Here's how the part is built. I have some questions about the finished solid (model axes, mm). Face numbers are marked on the shaded views. Give positions to 0.01 mm unless a question says otherwise; leave off trailing zeros. Loops run counter-clockwise (first coordinate to the right, second up) from the corner with the lowest first, then second, coordinate; pieces in that order, holes last.
Q1. I'm going to push flat-ended pins straight in: P1, Ø2.5, axis at x = 0, y = 0, coming from the +Z side; P2, Ø1.5, axis at x = 2, z = 0.5, coming from the -Y side. Where does each tip first touch, or does it pass through?
Q2. Suppose I cut it at D-D (z = 2.1). List the corners of the cut face in (x, y) for me, and give its area (3 significant figures).
Q3. Thinking about a two-plate mould opening in X: for the marked faces 1, 2 and 3, which applies, pulls with the +X half, pulls with the -X half, needs draft (parallel to the pull), parting line crosses it, or undercut?
Q4. Suppose I cut it at C-C (z = 1.25). List the corners of the cut face in (x, y) for me, and give its area (3 significant figures).
Q5. Suppose I cut it at A-A (y = 0). List the corners of the cut face in (x, z) for me, and give its area (3 significant figures).
Q6. I need wall thicknesses on probe 1 along Y at (x, z) = (0, 0.4); probe 2 along Y at (x, z) = (-2, 2); probe 3 along Z at (x, y) = (-2, -1). Which ranges of each line are inside material? Lowest first, please.
```python
from build123d import *

# Parameters (mm, degrees)
SKETCH_1_R      = 8
EXTRUDE_1_DEPTH = 2.5
CHAMFER_1_SIZE  = 1


with BuildPart() as part:
    # Эскиз1 → Бобышка-Вытянуть1 (new body)
    with BuildSketch(Plane.XY):
        Circle(SKETCH_1_R)
    extrude(amount=EXTRUDE_1_DEPTH)

    # Фаска1
    chamfer_1_edges = [part.edges().sort_by_distance(p)[0] for p in [
        (-8, 0, 2.5),
    ]]
    chamfer(chamfer_1_edges, length=CHAMFER_1_SIZE)

    # Эскиз4 → Зенковка для винта с полупотайной головкой M31 (revolve, cut)
    with BuildSketch(Plane(origin=(0, 0, 2.5), x_dir=(0, -1, 0), z_dir=(1, 0, 0))):
        Polygon((0, 0), (0, 2.5), (1.7, 2.5), (1.7, 1.45), (3.15, 0), align=None)
    revolve(axis=Axis((0, 0, 8.85), (0, 0, -1)), mode=Mode.SUBTRACT)


solid = part.part
```
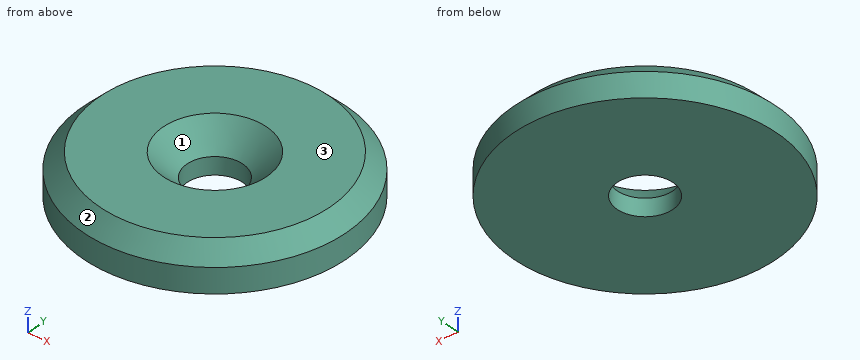
Solutions:
1. P1: passes through
1. P2: stops at y = -7.9
2. outline: circle Ø14.8 at (0, 0); hole circle Ø5.5 at (0, 0)
2. area: 148 mm2
3. face 1: undercut
3. face 2: parting line crosses it
3. face 3: needs draft
4. outline: circle Ø16 at (0, 0); hole circle Ø3.8 at (0, 0)
4. area: 190 mm2
5. outline: (-8, 0) - (-1.7, 0) - (-1.7, 1.05) - (-3.15, 2.5) - (-7, 2.5) - (-8, 1.5) - close; (1.7, 0) - (8, 0) - (8, 1.5) - (7, 2.5) - (3.15, 2.5) - (1.7, 1.05) - close
5. area: 28.4 mm2
6. probe 1: y = -8 to -1.7, 1.7 to 8
6. probe 2: y = -7.23 to -1.74, 1.74 to 7.23
6. probe 3: z = 0 to 1.59
